Read the model definition and answer for the solid it produces. Units are mm, in the model's axes. Face numbers are marked on the shaded views. A direction names the side the tool comes from. Coordinates: 2 decimals unless noted, no trailing zeros. Write each loop counter-clockwise with the first axis right and the second up, starting at its lowest first coordinate (ties: lowest second). Pieces come first, ordered by that corner, then holes.
(1) The part is cut by section C-C, the plane x = 25.5. Determine the outline of the cut face in (y, z) (3 decimals).
(2) The part is cut by section A-A, the plane z = 0. Determine the outline of the cut face in (x, y).
(3) Determine the mould class of the marked faces 4, 5 and 6 for opening direction X: pulls with the +X half, pulls with the -X half, needs draft (parallel to the pull), parting line crosses it, or undercut.
(4) Given pin 1 (4.5 mm diameter, centred on y = -12.7, z = 0, fed in from +X); pin 2 (1.5 mm diameter, centred on y = -14, z = 21.5, fed in from +X); pin 3 (2 mm diameter, centred on x = 28.5, z = 19, fed in from -Y), each flat-ended and moving along its own axis, determine where each tip first touches the part or whether it passes through.
(5) Which of the six approach directions +Z, -Z, +X, -X, +Y, -Y give full straight-line access (tool end or side, diameter ignored) to the marked faces 1, 2 and 3?
(6) Straight lines are drawn through the part: line 1 along Y through (x, z) = (1, 0); line 2 along Z through (x, y) = (4.5, -25.4) (3 decimals); line 3 along Z through (x, y) = (10, -22.5) (3 decimals). For each, find the intervals that lie inside material, in ascending order.
Autodesk Inventor part; units mm, degrees
ref_plane "YZ Plane" through (0, 0, 0) normal (1, 0, 0) x (0, 1, 0)
ref_plane "XZ Plane" through (0, 0, 0) normal (0, 1, 0) x (-1, 0, 0)
ref_plane "XY Plane" through (0, 0, 0) normal (0, 0, 1) x (1, 0, 0)
sketch "Sketch1" plane through (0, 0, 0) normal (0, 0, 1) x (1, 0, 0)
  line L0 (0, 0) -> (50.8, 0)
  line L1 (50.8, 0) -> (50.8, -6.35)
  line L2 (50.8, -6.35) -> (6.35, -6.35)
  line L3 (6.35, -6.35) -> (6.35, -38.1)
  line L4 (6.35, -38.1) -> (0, -38.1)
  line L5 (0, -38.1) -> (0, 0)
  dimension "d0" = 50.8
  dimension "d1" = 38.1
  dimension "d2" = 6.35
  dimension "d3" = 6.35
extrude "Extrusion1" add sketch "Sketch1" along normal mid plane 69.85
sketch "Sketch2" plane through (0, 0, 34.925) normal (0, 1, 0) x (1, 0, 0)
  line L0 (0, 69.85) -> (0, 0) construction
  line L1 (50.8, 0) -> (0, 0) construction
  line L2 (50.8, 69.85) -> (50.8, 0) construction
  line L3 (0, 69.85) -> (50.8, 69.85) construction
  circle A0 centre (28.575, 34.925) radius 11.2522
  line L4 (0, 0) -> (0, 69.85) construction
  line L5 (6.35, 69.85) -> (6.35, 0) construction
  line L6 (6.35, 69.85) -> (6.35, 0) construction
  line L7 (6.35, 69.85) -> (6.35, 0) construction
  line L8 (6.35, 69.85) -> (50.8, 69.85) construction
  line L9 (41.525, 36.525) -> (41.525, 33.325) construction
  line L10 (41.525, 36.525) -> (39.7129, 36.525) construction
  line L11 (41.525, 33.325) -> (39.7129, 33.325) construction
  line L12 (36.5315, 26.9685) -> (44.488, 34.925)
  line L13 (44.488, 34.925) -> (36.5315, 42.8815)
  line L14 (36.5315, 42.8815) -> (39.8272, 42.8815)
  line L15 (39.8272, 42.8815) -> (39.8272, 26.9685)
  line L16 (39.8272, 26.9685) -> (36.5315, 26.9685)
  line L17 (36.5315, 26.9685) -> (36.5315, 42.8815) construction
  point P0 (0, 34.925)
  point P1 (0, 34.925)
  point P2 (28.575, 69.85)
  point P3 (41.525, 34.925)
  point P4 (39.8272, 34.925)
  point P5 (39.8272, 39.5858)
  point P6 (39.8272, 30.2642)
  dimension "d6" = 22.5044
  dimension "d16" = 3.2
  dimension "d17" = 12.95
sketch "Sketch3" plane through (0, -38.1, 34.925) normal (-1, 0, 0) x (0, 0, 1)
  line L0 (0, 0) -> (-69.85, 0) construction
  line L1 (0, 38.1) -> (0, 0) construction
  line L2 (-69.85, 38.1) -> (0, 38.1) construction
  line L3 (-69.85, 0) -> (-69.85, 38.1) construction
  line L4 (-9.525, 25.4) -> (-60.325, 25.4) construction
  line L5 (-60.325, 25.4) -> (-60.325, 12.7) construction
  line L6 (-60.325, 12.7) -> (-9.525, 12.7) construction
  line L7 (-9.525, 12.7) -> (-9.525, 25.4) construction
  line L8 (-9.525, 25.4) -> (-60.325, 12.7) construction
  line L9 (-60.325, 25.4) -> (-9.525, 12.7) construction
  point P0 (-34.925, 38.1)
  point P1 (-34.925, 19.05)
  point P2 (-34.925, 38.1)
  point P3 (0, 19.05)
  point P4 (-34.925, 12.7)
  point P5 (-34.925, 25.4)
  dimension "d7" = 50.8
  dimension "d8" = 12.7
hole "Hole1" at (0, -12.7, -25.4) at (0, -25.4, -25.4) at (0, -25.4, 25.4) at (0, -12.7, 25.4) direction (1, 0, 0) diameter 5.1054 end through all
extrude "Extrusion2" cut sketch "Sketch2" against normal through all contours A0 | L15 L12 A0 | A0 L13 L15
fillet "Fillet1" [suppressed]
fillet "Fillet2" radius 12.7 2 edges at (50.8, -3.175, -34.925) (50.8, -3.175, 34.925)
fillet "Fillet3" radius 6.35 2 edges at (3.175, -38.1, -34.925) (3.175, -38.1, 34.925)
sketch "Sketch5" plane through (0, 0, -34.925) normal (0, 0, -1) x (-1, 0, 0)
  line L0 (0, -31.75) -> (-6.35, -31.75) construction
  line L1 (0, -31.75) -> (0, 0) construction
  line L2 (0, 0) -> (-38.1, 0) construction
  line L3 (-38.1, -6.35) -> (-38.1, 0) construction
  line L4 (-38.1, -6.35) -> (-6.35, -6.35) construction
  line L5 (-6.35, -6.35) -> (-6.35, -31.75) construction
  line L6 (-38.1, -6.35) -> (-6.35, -31.75)
  line L7 (-6.35, -6.35) -> (-6.35, -31.75)
  line L8 (-6.35, -27.9527) -> (-6.35, -22.8473) construction
  line L9 (-6.35, -6.35) -> (-38.1, -6.35)
  line L10 (-17.3228, -6.35) -> (-17.3228, -6.35) construction
  point P0 (-36.5315, -6.35)
extrude "Extrusion3" add sketch "Sketch5" against normal blind 3
mirror "Mirror1" about plane through (0, 0, 0) normal (0, 0, 1) of "Extrusion3"
fillet "Fillet4" radius 6.35 2 edges at (22.225, -6.35, 31.925) (22.225, -6.35, -31.925)
sketch "Sketch6" plane through (6.35, -38.1, 28.575) normal (1, 0, 0) x (0, 0, -1)
  line L0 (43.4887, 15.24) -> (13.6613, 15.24) construction
  line L1 (13.6613, 15.24) -> (13.6613, 22.86) construction
  line L2 (13.6613, 22.86) -> (43.4887, 22.86) construction
  line L3 (43.4887, 22.86) -> (43.4887, 15.24) construction
  line L4 (50.8, 38.1) -> (6.35, 38.1) construction
  circle A0 centre (3.175, 25.4) radius 2.5527 construction
  circle A1 centre (3.175, 12.7) radius 2.5527 construction
  line L5 (3.175, 25.4) -> (3.175, 12.7) construction
  point P0 (28.575, 38.1)
  point P1 (28.575, 15.24)
  point P2 (28.575, 38.1)
  point P3 (43.4887, 19.05)
  point P4 (3.175, 19.05)
  point P5 (13.6613, 19.05)
  point P6 (28.575, 22.86)
  point P7 (28.575, 38.1)
  dimension "d0" = 50.8
  dimension "d1" = 38.1
  dimension "d2" = 6.35
  dimension "d3" = 6.35
  dimension "d29" = 7.62
  dimension "d30" = 29.8274
extrude "Extrusion4" [suppressed]
sketch "Sketch7" plane through (6.35, -38.1, 28.575) normal (1, 0, 0) x (0, 0, -1)
  point P0 (28.575, 38.1)
sketch "Sketch8" plane through (0, 0, -34.925) normal (-1, 0, 0) x (0, 0, 1)
  arc A0 (0, -31.75) -> (6.35, -38.1) centre (6.35, -31.75) ccw construction
  line L0 (0, -31.75) -> (0, 0) construction
  line L1 (0, 0) -> (69.85, 0) construction
  line L2 (69.85, 0) -> (69.85, -31.75) construction
  arc A1 (63.5, -38.1) -> (69.85, -31.75) centre (63.5, -31.75) ccw construction
  line L3 (63.5, -38.1) -> (6.35, -38.1) construction
  circle A2 centre (60.325, -25.4) radius 2.5527
  circle A3 centre (9.525, -12.7) radius 2.5527
  circle A4 centre (9.525, -25.4) radius 2.5527
  circle A5 centre (60.325, -12.7) radius 2.5527
  line L4 (60.325, -25.4) -> (9.525, -25.4) construction
  line L5 (9.525, -25.4) -> (9.525, -12.7) construction
  line L6 (9.525, -12.7) -> (60.325, -12.7) construction
  line L7 (60.325, -12.7) -> (60.325, -25.4) construction
  point P0 (34.925, 0)
  point P1 (34.925, -25.4)
  point P2 (34.925, -12.7)
hole "Hole2" at (0, -25.4, 0) at (0, -12.7, 0) direction (1, 0, 0) diameter 5.1054 end through all
extrude "Extrusion5" add sketch "Sketch8" against normal up to surface (6.35 mm away)
properties part number "rsl mount" material "ABS Plastic"
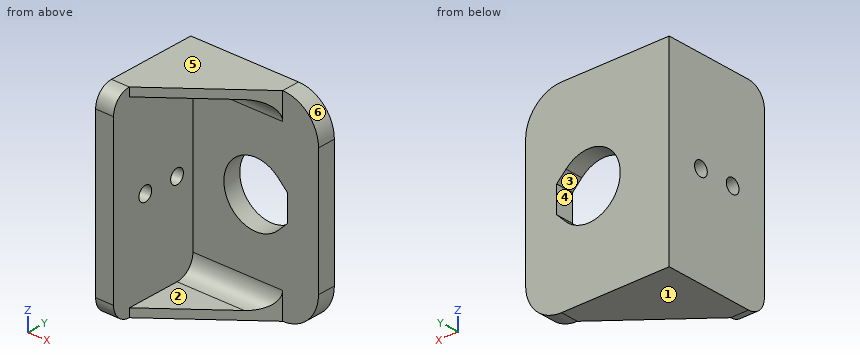
Computed:
1. outline: (-16.43, -34.925) - (0, -34.925) - (0, -10.824) - (-6.35, -10.824) - (-6.35, -25.575) arc R6.35 cw to (-12.7, -31.925) - (-16.43, -31.925) - close; (-16.43, 31.925) - (-12.7, 31.925) arc R6.35 cw to (-6.35, 25.575) - (-6.35, 10.824) - (0, 10.824) - (0, 34.925) - (-16.43, 34.925) - close
2. outline: (0, -38.1) - (6.35, -38.1) - (6.35, -27.95) - (0, -27.95) - close; (0, -22.85) - (6.35, -22.85) - (6.35, -15.25) - (0, -15.25) - close; (0, -10.15) - (6.35, -10.15) - (6.35, -6.35) - (17.32, -6.35) - (17.32, 0) - (0, 0) - close; (39.83, -6.35) - (50.8, -6.35) - (50.8, 0) - (39.83, 0) - close
3. face 4: undercut
3. face 5: needs draft
3. face 6: pulls with the +X half
4. pin 1: passes through
4. pin 2: stops at x = 6.35
4. pin 3: stops at y = -6.35
5. face 1: -Z, +X, -X, +Y, -Y
5. face 2: +X, -Y
5. face 3: +Y, -Y
6. line 1: y = -38.1 to -27.95, -22.85 to -15.25, -10.15 to 0
6. line 2: z = -34.925 to -2.553, 2.553 to 34.925
6. line 3: z = -34.925 to -31.925, 31.925 to 34.925
